Work out the finished part from the listing and answer in its coordinate system (mm). A direction names the side the tool comes from. Give positions to 0.01 mm unless a question says otherwise; leave off trailing zeros. Loops run counter-clockwise (first coordinate to the right, second up) from the corner with the lowest first, then second, coordinate; pieces in that order, holes last. Notation, with made-up numbers: M 23.5,-32.5 L 73.5,-32.5 A30 cw 73.5,1.5 Z; hole C -2.5,-6.5 d9. An arc over 180 degrees is marked long. Answer in a Markdown table with one row per item. Add a question column.
from build123d import *

# Parameters (mm, degrees)
SKETCH2_R                = 2.0399375
SKETCH2_R_2              = 1.5319375
BOSS_EXTRUDE1_DEPTH      = 1.5875
BOSS_EXTRUDE3_DEPTH      = 1.5875
BOSS_EXTRUDE3_DEPTH_BACK = 1.5875
SKETCH2_4_R              = 1.5319375
FILLET1_R                = 1.5875


with BuildPart() as part:
    # Sketch2 → Boss-Extrude1 (new body)
    with BuildSketch(Plane.XY):
        with BuildLine():
            ThreePointArc((0, 5.55625), (-5.113202022, 2.174184709), (-4.001636229, -3.854714199))
            ThreePointArc((-4.001636229, -3.854714199), (-3.061446645, -5.685103398), (-3.287058415, -7.730434766))
            ThreePointArc((-3.287058415, -7.730434766), (0, -12.7), (3.287058415, -7.730434766))
            ThreePointArc((3.287058415, -7.730434766), (3.061446641, -5.685103418), (4.0016362, -3.854714229))
            ThreePointArc((4.0016362, -3.854714229), (5.152960566, -2.078199091), (5.55625, 0))
            Line((5.55625, 0), (23.01875, 0))
            ThreePointArc((23.01875, 0), (23.422039385, -2.07819897), (24.573363619, -3.854714041))
            ThreePointArc((24.573363619, -3.854714041), (25.513553344, -5.685103337), (25.287941547, -7.730434854))
            ThreePointArc((25.287941547, -7.730434854), (28.575000048, -12.7), (31.862058415, -7.730434766))
            ThreePointArc((31.862058415, -7.730434766), (31.636446655, -5.685103342), (32.576636308, -3.854714117))
            ThreePointArc((32.576636308, -3.854714117), (34.13125, -7.3e-08), (32.576636409, 3.854714012))
            ThreePointArc((32.576636409, 3.854714012), (31.636446674, 5.685103241), (31.862058392, 7.730434711))
            ThreePointArc((31.862058392, 7.730434711), (29.288207306, 12.628071622), (25.003125, 9.128125))
            ThreePointArc((25.003125, 9.128125), (23.956947034, 6.602427966), (21.43125, 5.55625))
            Line((21.43125, 5.55625), (0, 5.55625))
        make_face()
        Circle(SKETCH2_R, mode=Mode.SUBTRACT)
        with Locations((28.575, 0)):
            Circle(SKETCH2_R, mode=Mode.SUBTRACT)
        with Locations((28.575, 9.128125)):
            Circle(SKETCH2_R_2, mode=Mode.SUBTRACT)
        with Locations((0, -9.128125)):
            Circle(SKETCH2_R, mode=Mode.SUBTRACT)
        with Locations((28.575, -9.128125)):
            Circle(SKETCH2_R, mode=Mode.SUBTRACT)
    extrude(amount=BOSS_EXTRUDE1_DEPTH)

    # Sketch2<4> → Boss-Extrude3 (add, two sides: drawn at the far end of the back side and taken through both)
    with BuildSketch(Plane.XY.offset(-BOSS_EXTRUDE3_DEPTH_BACK)):
        with Locations((28.575, 9.128125)):
            Circle(SKETCH2_4_R)
    extrude(amount=BOSS_EXTRUDE3_DEPTH + BOSS_EXTRUDE3_DEPTH_BACK)

    # Fillet1
    fillet1_edges = [part.edges().sort_by_distance(p)[0] for p in [
        (23.01875, 0, 0.79375),
        (5.55625, 0, 0.79375),
    ]]
    fillet(fillet1_edges, radius=FILLET1_R)


solid = part.part
(1) Which of the six approach directions +Z, -Z, +X, -X, +Y, -Y give full straight-line access (tool end or side, diameter ignored) to faces 1 (the face through (1.884, -0.781, 0.783)), 2 (the face through (5.96, -0.36, 0.8)), 3 (the face through (11, 5.556, 1))?
(2) Section B-B, the plane y = -5.75 is taken. Determine the outline of the cut face in (x, z), and give its area (3 significant figures).
(3) Section A-A, the plane z = 0.45 is taken. Determine the outline of the cut face in (x, y) (1 decimal), and give its area (3 significant figures).
(4) The mould has two halves that part along Y. Classify faces 4 (the face through (30.036, 9.588, -0.805)), 5 (the face through (30.52, 0.61, 0.78)), 6 (the face through (4.88, -2.66, 0.78)): pulls with the +Y half, pulls with the -Y half, needs draft (parallel to the pull), parting line crosses it, or undercut.
(5) Consider line 1 along Y through (x, z) = (27, 1.45); line 2 along Z through (x, y) = (29.5, 7.25); line 3 along Y through (x, z) = (12.5, 0.5). Determine where each line is inside the solid, lowest interval first. Write a range as from..to.
(6) Section D-D, the plane x = 17 is taken. Determine the outline of the cut face in (y, z).
(7) Section C-C, the plane y = -10.75 is taken. Determine the outline of the cut face in (x, z).
(8) Each of these flat-tipped pins is pushed along its axis until it touches: P1, Ø5.5, axis at x = 0, y = -9.13, coming from the -Z side; P2, Ø1.7, axis at x = 16, z = 0.5, coming from the -Y side; P3, Ø0.5, axis at x = 15, z = 1, coming from the +Y side. Where does it stop, or does it pass through?
Numbers:
| question | item | result |
|---|---|---|
| 1 | face 1 | +Z, -Z |
| 1 | face 2 | +Z, -Z, -Y |
| 1 | face 3 | +Z, -Z, -X, +Y |
| 2 | outline | M -3.05,0 L 3.05,0 L 3.05,1.59 L -3.05,1.59 Z; M 25.52,0 L 31.63,0 L 31.63,1.59 L 25.52,1.59 Z |
| 2 | area | 19.4 mm² |
| 3 | outline | M -4,-3.9 A3.6 cw -3.3,-7.7 A3.6 ccw long 3.3,-7.7 A3.6 cw 4,-3.9 A5.6 ccw 5.4,-1.2 A1.6 cw 7,0 L 21.6,0 A1.6 cw 23.2,-1.2 A5.6 ccw 24.6,-3.9 A3.6 cw 25.3,-7.7 A3.6 ccw long 31.9,-7.7 A3.6 cw 32.6,-3.9 A5.6 ccw 32.6,3.9 A3.6 cw 31.9,7.7 A3.6 ccw long 25,9.1 A3.6 cw 21.4,5.6 L 0,5.6 A5.6 ccw Z; hole C 0,-9.1 d4.1; hole C 0,0 d4.1; hole C 28.6,-9.1 d4.1; hole C 28.6,0 d4.1 |
| 3 | area | 392 mm² |
| 4 | face 4 | parting line crosses it |
| 4 | face 5 | undercut |
| 4 | face 6 | pulls with the -Y half |
| 5 | line 1 | y = -12.33..-10.42, -7.83..-1.3, 1.3..12.33 |
| 5 | line 2 | z = 0..1.59 |
| 5 | line 3 | y = 0..5.56 |
| 6 | outline | M 0,0 L 5.56,0 L 5.56,1.59 L 0,1.59 Z |
| 7 | outline | M -3.18,0 L -1.24,0 L -1.24,1.59 L -3.18,1.59 Z; M 1.24,0 L 3.18,0 L 3.18,1.59 L 1.24,1.59 Z; M 25.39,0 L 27.34,0 L 27.34,1.59 L 25.39,1.59 Z; M 29.81,0 L 31.76,0 L 31.76,1.59 L 29.81,1.59 Z |
| 8 | P1 | stops at z = 0 |
| 8 | P2 | stops at y = 0 |
| 8 | P3 | stops at y = 5.56 |
